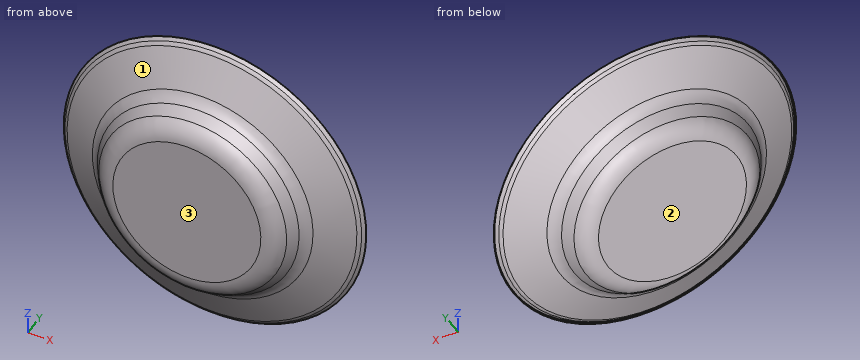
```python
from build123d import *


with BuildPart() as part:
    # Sketch1 → Revolve-Thin2 (revolve)
    with BuildSketch(Plane.XY, mode=Mode.PRIVATE) as revolve_thin2_sk:
        with BuildLine():
            Line((0, 0), (-30.323190326, 0))
            ThreePointArc((-30.323190326, 0), (-34.9291722, 1.123912406), (-38.499810041, 4.243013806))
            Line((-38.499810041, 4.243013806), (-41.339639807, 8.276410321))
            ThreePointArc((-41.339639807, 8.276410321), (-43.060923254, 10.156742614), (-45.201704548, 11.540766343))
            Line((-45.201704548, 11.540766343), (-59.366864821, 18.315408212))
            ThreePointArc((-59.366864821, 18.315408212), (-60.097449611, 18.744382189), (-60.74512124, 19.290545415))
            Line((-60.74512124, 19.290545415), (-61.963641622, 20.509065797))
            Line((-61.963641622, 20.509065797), (-61.610088232, 20.862619188))
            Line((-61.610088232, 20.862619188), (-60.391567849, 19.644098805))
            ThreePointArc((-60.391567849, 19.644098805), (-59.808663383, 19.152551902), (-59.151137072, 18.766475323))
            Line((-59.151137072, 18.766475323), (-44.9859768, 11.991833454))
            ThreePointArc((-44.9859768, 11.991833454), (-42.73815644, 10.538608538), (-40.930808821, 8.56425963))
            Line((-40.930808821, 8.56425963), (-38.090979055, 4.530863116))
            ThreePointArc((-38.090979055, 4.530863116), (-34.698873107, 1.567716786), (-30.323190326, 0.5))
            Line((-30.323190326, 0.5), (0, 0.5))
            Line((0, 0.5), (0, 0))
        make_face()
    revolve(revolve_thin2_sk.sketch.rotate(Axis((0, 28.049813209, 0), (0, -1, 0)), 270), axis=Axis((0, 28.049813209, 0), (0, -1, 0)))


solid = part.part
```
Geometry check sheet. Reference: the model listing, model coordinates, mm. Face numbers are marked on the shaded views. Coordinates: 2 decimals unless noted, no trailing zeros. Loops run counter-clockwise (first coordinate to the right, second up) from the corner with the lowest first, then second, coordinate; pieces in that order, holes last.
Item 1: Release check for a two-part mould opening along Z. For the marked faces 1, 2 and 3 record: released by +Z, released by -Z, zero draft, split by the parting line, or undercut.
Item 2: Sectioned sample at C-C, the plane y = 6.5. Record the boundary of the cut face in (x, z).
Item 3: Thickness scan on line 1 (X direction, y = 18.5, z = -9); line 2 (Z direction, x = 11, y = 16.25); line 3 (X direction, y = 3, z = 26.5). Record the ranges inside material, lowest first.
Item 4: Go/stop test with flat-tipped pins: pin 1 Ø18 at (x, z) = (1.5, 5) entering from +Y; pin 2 Ø5 at (y, z) = (14, -4) entering from -X; pin 3 Ø2 at (x, y) = (-12, 7.5) entering from +Z. Record where each tip stops, or that it passes through.
Item 5: Sectioned sample at A-A, the plane x = 0. Record the boundary of the cut face in (y, z).
Item 6: Sectioned sample at B-B, the plane z = 0. Record the boundary of the cut face in (x, y).
Check result:
1. face 1: split by the parting line
1. face 2: undercut
1. face 3: zero draft
2. outline: circle Ø80.18 at (0, 0); hole circle Ø78.95 at (0, 0)
3. line 1: x = -59.03 to -57.9, 57.9 to 59.03
3. line 2: z = -53.94 to -52.75, 52.75 to 53.94
3. line 3: x = -26.48 to -25.46, 25.46 to 26.48
4. pin 1: stops at y = 0.5
4. pin 2: stops at x = -55.43
4. pin 3: stops at z = 39.78
5. outline: (0, -30.32) arc R10 ccw to (4.24, -38.5) - (8.28, -41.34) arc R10 cw to (11.54, -45.2) - (18.32, -59.37) arc R5 ccw to (19.29, -60.75) - (20.51, -61.96) - (20.86, -61.61) - (19.64, -60.39) arc R4.5 cw to (18.77, -59.15) - (11.99, -44.99) arc R10.5 ccw to (8.56, -40.93) - (4.53, -38.09) arc R9.5 cw to (0.5, -30.32) - (0.5, 30.32) arc R9.5 cw to (4.53, 38.09) - (8.56, 40.93) arc R10.5 ccw to (11.99, 44.99) - (18.77, 59.15) arc R4.5 cw to (19.64, 60.39) - (20.86, 61.61) - (20.51, 61.96) - (19.29, 60.75) arc R5 ccw to (18.32, 59.37) - (11.54, 45.2) arc R10 cw to (8.28, 41.34) - (4.24, 38.5) arc R10 ccw to (0, 30.32) - close
6. outline: (-61.96, 20.51) - (-60.75, 19.29) arc R5 ccw to (-59.37, 18.32) - (-45.2, 11.54) arc R10 cw to (-41.34, 8.28) - (-38.5, 4.24) arc R10 ccw to (-30.32, 0) - (30.32, 0) arc R10 ccw to (38.5, 4.24) - (41.34, 8.28) arc R10 cw to (45.2, 11.54) - (59.37, 18.32) arc R5 ccw to (60.75, 19.29) - (61.96, 20.51) - (61.61, 20.86) - (60.39, 19.64) arc R4.5 cw to (59.15, 18.77) - (44.99, 11.99) arc R10.5 ccw to (40.93, 8.56) - (38.09, 4.53) arc R9.5 cw to (30.32, 0.5) - (-30.32, 0.5) arc R9.5 cw to (-38.09, 4.53) - (-40.93, 8.56) arc R10.5 ccw to (-44.99, 11.99) - (-59.15, 18.77) arc R4.5 cw to (-60.39, 19.64) - (-61.61, 20.86) - close
